from build123d import *

# Parameters (mm, degrees)
SKETCH1_W                               = 56
SKETCH1_H                               = 25
BOSS_EXTRUDE1_DEPTH                     = 14
CBORE_FOR_M5_HEX_HEAD_BOLT1_D           = 5.5
CBORE_FOR_M5_HEX_HEAD_BOLT1_CBORE_D     = 11
CBORE_FOR_M5_HEX_HEAD_BOLT1_CBORE_DEPTH = 5
SKETCH9_W                               = 25
SKETCH9_H                               = 8
CUT_EXTRUDE2_DEPTH                      = 3
SKETCH8_W                               = 5.8
SKETCH8_H                               = 2
CUT_EXTRUDE1_DEPTH                      = 10
F_3_0MM_DOWEL_HOLE1_D                   = 3.3
F_3_0MM_DOWEL_HOLE1_DEPTH               = 8
F_3_0MM_DOWEL_HOLE1_TIP                 = 0.991420021
FILLET1_R                               = 2
CHAMFER2_SIZE                           = 3


# Some blends are built 0.0001 mm under size
with BuildPart() as part:
    # Sketch1 → Boss-Extrude1 (new, symmetric)
    with BuildSketch(Plane.XY):
        with Locations((-28, 12.5)):
            Rectangle(SKETCH1_W, SKETCH1_H)
    extrude(amount=BOSS_EXTRUDE1_DEPTH, both=True)

    # CBORE for M5 Hex Head Bolt1 (through all)
    with Locations(Plane.XY.offset(14)):
        with Locations((-48, 10)):
            CounterBoreHole(CBORE_FOR_M5_HEX_HEAD_BOLT1_D / 2, CBORE_FOR_M5_HEX_HEAD_BOLT1_CBORE_D / 2, CBORE_FOR_M5_HEX_HEAD_BOLT1_CBORE_DEPTH)

    # Sketch9 → Cut-Extrude2 (cut)
    with BuildSketch(Plane(origin=(0, 25, 0), x_dir=(1, 0, 0), z_dir=(0, 1, 0))):
        with Locations((-31.5, 10)):
            Rectangle(SKETCH9_W, SKETCH9_H)
        with Locations((-31.5, -10)):
            Rectangle(SKETCH9_W, SKETCH9_H)
    extrude(amount=-CUT_EXTRUDE2_DEPTH, mode=Mode.SUBTRACT)

    # Sketch8 → Cut-Extrude1 (cut)
    with BuildSketch(Plane.ZY.offset(56)):
        with Locations((-9.5, 21)):
            Rectangle(SKETCH8_W, SKETCH8_H)
        with Locations((9.5, 21)):
            Rectangle(SKETCH8_W, SKETCH8_H)
    extrude(amount=-CUT_EXTRUDE1_DEPTH, mode=Mode.SUBTRACT)

    # Mirror1: part across plane


with BuildPart() as part_1:
    add(part.part)
    add(part.part.mirror(Plane(origin=(0, 25, 14), x_dir=(0, 0, 1), z_dir=(-1, 0, 0))))

    # Ø3.0mm Dowel Hole1
    with Locations(Plane(origin=(0, 25, 0), x_dir=(1, 0, 0), z_dir=(0, 1, 0))):
        with Locations((49.74, 9.5), (-49.74, -9.5), (-49.74, 9.5), (49.74, -9.5)):
            Hole(F_3_0MM_DOWEL_HOLE1_D / 2, depth=F_3_0MM_DOWEL_HOLE1_DEPTH)
            with Locations((0, 0, -(F_3_0MM_DOWEL_HOLE1_DEPTH + F_3_0MM_DOWEL_HOLE1_TIP / 2))):  # 118° drill point
                Cone(0, F_3_0MM_DOWEL_HOLE1_D / 2, F_3_0MM_DOWEL_HOLE1_TIP, mode=Mode.SUBTRACT)

    # Fillet1
    # the kernel refuses this fillet: 2 mm, written as the material it takes off along each edge
    with BuildSketch(Plane(origin=(-56, 30, -14), x_dir=(0, 0, 1), z_dir=(0, -1, 0)), Plane(origin=(56, 30, -14), x_dir=(-1, 0, 0), z_dir=(0, -1, 0))) as fillet1_piece_1:
        with BuildLine():
            CenterArc((FILLET1_R, -FILLET1_R), FILLET1_R, 90, 90)
            Line((0, -FILLET1_R), (0, 0))
            Line((0, 0), (FILLET1_R, 0))
        make_face()
    extrude(amount=35, mode=Mode.SUBTRACT)
    with BuildSketch(Plane(origin=(-56, 30, 14), x_dir=(0, 0, -1), z_dir=(0, -1, 0)), Plane(origin=(56, 30, 14), x_dir=(-1, 0, 0), z_dir=(0, -1, 0))) as fillet1_piece_2:
        with BuildLine():
            CenterArc((FILLET1_R, FILLET1_R), FILLET1_R, 180, 90)
            Line((0, FILLET1_R), (0, 0))
            Line((0, 0), (FILLET1_R, 0))
        make_face()
    extrude(amount=35, mode=Mode.SUBTRACT)

    # Chamfer2
    chamfer2_edges = [part_1.edges().sort_by_distance(p)[0] for p in [
        (-31.5, 22, 6),
        (31.5, 22, 6),
        (-31.5, 22, -6),
        (31.5, 22, -6),
    ]]
    chamfer(chamfer2_edges, length=CHAMFER2_SIZE - 0.0001)  # a hair under: the kernel refuses the full size


solid = part_1.part
Could you check a few things on this model? Use its own coordinates, in mm. A direction names the side the tool comes from. Give positions to 0.01 mm unless a question says otherwise; leave off trailing zeros. Write each loop counter-clockwise with the first axis right and the second up, starting at its lowest first coordinate (ties: lowest second). Pieces come first, ordered by that corner, then holes. Notation, with made-up numbers: (10.25, 57) -> (56.25, 57) arc R25 ccw to (56.25, 94) -> close; hole circle Ø5 at (8.5, 29). An arc over 180 degrees is marked (long way). Answer as a JSON object with one key per item and string values.
Q1. Which directions (+Z, -Z, +X, -X, +Y, -Y) give clear straight access to the entire face, cutting with the end or side of a thin tool? Please do faces 1 (the flat face through (52, 22, -10)), 2 (the cylindrical face through (-53.495, 10.242, 11.535)), 3 (the cylindrical face through (-51.264, 23.479, 10.132)), 4 (the flat face through (32, 22, 11)).
Taken from the geometry:
{"face 1": "+X", "face 2": "+Z", "face 3": "+Y", "face 4": "+Z, +Y"}
Q2. We'd pull the mould along Y, two halves only. Please class faces 5 (the flat face through (32, 23, -8)), 6 (the flat face through (-51, 21, 6.6)), 7 (the cylindrical face through (48.216, 18.479, -8.868)): released by +Y, released by -Y, zero draft, split by the parting line, or undercut.
Taken from the geometry:
{"face 5": "released by +Y", "face 6": "undercut", "face 7": "zero draft"}
Q3. Suppose I cut it at A-A on z = -1. Write out the boundary of the cut face in (x, y), then the cut area to 3 significant figures.
Taken from the geometry:
{"outline": "(-56, 0) -> (56, 0) -> (56, 25) -> (-56, 25) -> close; hole circle Ø5.5 at (-48, 10); hole circle Ø5.5 at (48, 10)", "area": "2,750 mm²"}
Q4. Will these pins go through, and if not, where does the flat tip stop? pin 1 Ø12.5 at (x, y) = (48, 10) entering from -Z; pin 2 Ø3 at (x, z) = (-49.74, -9.5) entering from +Y; pin 3 Ø2.5 at (x, z) = (-49.74, 9.5) entering from +Y.
Taken from the geometry:
{"pin 1": "stops at z = -14", "pin 2": "stops at y = 16.91", "pin 3": "stops at y = 16.76"}
Q5. Please list where these lines run through material, in increasing order: L1, parallel to X at y = 23.85, z = -9.5; L2, parallel to Z at x = -49.74, y = 23.85; L3, parallel to X at y = 19, z = -9.5.
Taken from the geometry:
{"L1": "x = -56 to -51.39, -48.09 to -44, -19 to 19, 44 to 48.09, 51.39 to 56", "L2": "z = -14 to -11.15, -7.85 to 7.85, 11.15 to 14", "L3": "x = -56 to -51.39, -48.09 to 48.09, 51.39 to 56"}
